Verification items for the finished model (mm, model axes). Face numbers are marked on the shaded views. A direction names the side the tool comes from. Give positions to 0.01 mm unless a question says otherwise; leave off trailing zeros. Loops run counter-clockwise (first coordinate to the right, second up) from the corner with the lowest first, then second, coordinate; pieces in that order, holes last. Notation, with made-up numbers: (77.5, -30) - (122.5, -30) arc R27 ccw to (122.5, 3) - close; hole circle Ø6 at (-25, 9). An arc over 180 degrees is marked (long way). Put each result on its own line as item: value. Start each with the question number.
```python
from build123d import *

# Parameters (mm, degrees)
SKETCH1_W            = 100
SKETCH1_H            = 16
BOSS_EXTRUDE1_DEPTH  = 3
SKETCH2_W            = 98
SKETCH2_H            = 14
CUT_EXTRUDE1_DEPTH   = 1
SKETCH5_W            = 20
SKETCH5_H            = 3
BOSS_EXTRUDE4_DEPTH  = 15
SKETCH6_W            = 20
SKETCH6_H            = 3
BOSS_EXTRUDE5_DEPTH  = 15
FILLET18_R           = 10
SKETCH7_W            = 3
SKETCH7_H            = 12
BOSS_EXTRUDE6_DEPTH  = 16
SKETCH8_W            = 6
SKETCH8_H            = 2
BOSS_EXTRUDE7_DEPTH  = 2
FILLET19_R           = 6
SKETCH10_W           = 60
SKETCH10_H           = 3
BOSS_EXTRUDE8_DEPTH  = 3
SKETCH11_W           = 60
SKETCH11_H           = 3
BOSS_EXTRUDE9_DEPTH  = 3
SKETCH12_W           = 0.95
SKETCH12_H           = 14
BOSS_EXTRUDE10_DEPTH = 3
SKETCH13_W           = 100
SKETCH13_H           = 0.95
BOSS_EXTRUDE11_DEPTH = 3
SKETCH14_W           = 0.95
SKETCH14_H           = 0.052088128
BOSS_EXTRUDE12_DEPTH = 3
SKETCH15_W           = 0.95
SKETCH15_H           = 0.047911872
SKETCH15_W_2         = 0.949734752
SKETCH15_H_2         = 0.052088128
BOSS_EXTRUDE13_DEPTH = 3
FILLET20_R           = 10
SKETCH17_W           = 98.1
SKETCH17_H           = 14.1
SKETCH17_W_2         = 97.1
SKETCH17_H_2         = 13.1
CUT_EXTRUDE2_DEPTH   = 4
SKETCH18_W           = 100
SKETCH18_H           = 16.05
SKETCH18_W_2         = 98
SKETCH18_H_2         = 14.05
CUT_EXTRUDE3_DEPTH   = 2


with BuildPart() as part:
    # Sketch1 → Boss-Extrude1 (new body)
    with BuildSketch(Plane(origin=(0, 0, 0), x_dir=(1, 0, 0), z_dir=(0, 1, 0))):
        with Locations((50, 8)):
            Rectangle(SKETCH1_W, SKETCH1_H)
    extrude(amount=BOSS_EXTRUDE1_DEPTH)

    # Sketch2 → Cut-Extrude1 (cut)
    with BuildSketch(Plane(origin=(0, 3, 0), x_dir=(1, 0, 0), z_dir=(0, 1, 0))):
        with Locations((50, 8)):
            Rectangle(SKETCH2_W, SKETCH2_H)
    extrude(amount=-CUT_EXTRUDE1_DEPTH, mode=Mode.SUBTRACT)

    # Sketch5 → Boss-Extrude4 (add)
    with BuildSketch(Plane.XY):
        with Locations((10, 1.5)):
            Rectangle(SKETCH5_W, SKETCH5_H)
        with Locations((90, 1.5)):
            Rectangle(SKETCH5_W, SKETCH5_H)
    extrude(amount=BOSS_EXTRUDE4_DEPTH)

    # Sketch6 → Boss-Extrude5 (add)
    with BuildSketch(Plane(origin=(0, 0, -16), x_dir=(-1, 0, 0), z_dir=(0, 0, -1))):
        with Locations((-90, 1.5)):
            Rectangle(SKETCH6_W, SKETCH6_H)
        with Locations((-10, 1.5)):
            Rectangle(SKETCH6_W, SKETCH6_H)
    extrude(amount=BOSS_EXTRUDE5_DEPTH)

    # Fillet18
    fillet18_edges = [part.edges().sort_by_distance(p)[0] for p in [
        (20, 1.5, 15),
        (0, 1.5, 15),
        (80, 1.5, 15),
        (100, 1.5, 15),
        (0, 1.5, -31),
        (20, 1.5, -31),
        (80, 1.5, -31),
        (100, 1.5, -31),
    ]]
    fillet(fillet18_edges, radius=FILLET18_R - 0.0001)  # a hair under: the kernel refuses the full size

    # Sketch7 → Boss-Extrude6 (add)
    with BuildSketch(Plane(origin=(0, 2, 0), x_dir=(1, 0, 0), z_dir=(0, 1, 0))):
        with Locations((95, 8)):
            Rectangle(SKETCH7_W, SKETCH7_H)
        with Locations((86, 8)):
            Rectangle(SKETCH7_W, SKETCH7_H)
        with Locations((77, 8)):
            Rectangle(SKETCH7_W, SKETCH7_H)
        with Locations((68, 8)):
            Rectangle(SKETCH7_W, SKETCH7_H)
        with Locations((59, 8)):
            Rectangle(SKETCH7_W, SKETCH7_H)
        with Locations((50, 8)):
            Rectangle(SKETCH7_W, SKETCH7_H)
        with Locations((41, 8)):
            Rectangle(SKETCH7_W, SKETCH7_H)
        with Locations((32, 8)):
            Rectangle(SKETCH7_W, SKETCH7_H)
        with Locations((23, 8)):
            Rectangle(SKETCH7_W, SKETCH7_H)
        with Locations((14, 8)):
            Rectangle(SKETCH7_W, SKETCH7_H)
        with Locations((5, 8)):
            Rectangle(SKETCH7_W, SKETCH7_H)
    extrude(amount=BOSS_EXTRUDE6_DEPTH)

    # Sketch8 → Boss-Extrude7 (add)
    with BuildSketch(Plane(origin=(0, 2, 0), x_dir=(1, 0, 0), z_dir=(0, 1, 0))):
        with Locations((90.5, 8)):
            Rectangle(SKETCH8_W, SKETCH8_H)
        with Locations((81.5, 8)):
            Rectangle(SKETCH8_W, SKETCH8_H)
        with Locations((72.5, 8)):
            Rectangle(SKETCH8_W, SKETCH8_H)
        with Locations((63.5, 8)):
            Rectangle(SKETCH8_W, SKETCH8_H)
        with Locations((54.5, 8)):
            Rectangle(SKETCH8_W, SKETCH8_H)
        with Locations((45.5, 8)):
            Rectangle(SKETCH8_W, SKETCH8_H)
        with Locations((36.5, 8)):
            Rectangle(SKETCH8_W, SKETCH8_H)
        with Locations((27.5, 8)):
            Rectangle(SKETCH8_W, SKETCH8_H)
        with Locations((18.5, 8)):
            Rectangle(SKETCH8_W, SKETCH8_H)
        with Locations((9.5, 8)):
            Rectangle(SKETCH8_W, SKETCH8_H)
    extrude(amount=BOSS_EXTRUDE7_DEPTH)

    # Fillet19
    fillet19_edges = [part.edges().sort_by_distance(p)[0] for p in [
        (95, 18, -2),
        (95, 18, -14),
        (86, 18, -2),
        (86, 18, -14),
        (77, 18, -2),
        (77, 18, -14),
        (68, 18, -2),
        (68, 18, -14),
        (59, 18, -2),
        (59, 18, -14),
        (50, 18, -2),
        (50, 18, -14),
        (41, 18, -2),
        (41, 18, -14),
        (32, 18, -2),
        (32, 18, -14),
        (23, 18, -14),
        (23, 18, -2),
        (14, 18, -2),
        (14, 18, -14),
        (5, 18, -2),
        (5, 18, -14),
    ]]
    fillet(fillet19_edges, radius=FILLET19_R - 0.0001)  # a hair under: the kernel refuses the full size

    # Sketch10 → Boss-Extrude8 (add)
    with BuildSketch(Plane(origin=(0, 0, -16), x_dir=(-1, 0, 0), z_dir=(0, 0, -1))):
        with Locations((-50, 1.5)):
            Rectangle(SKETCH10_W, SKETCH10_H)
    extrude(amount=BOSS_EXTRUDE8_DEPTH)

    # Sketch11 → Boss-Extrude9 (add)
    with BuildSketch(Plane.XY):
        with Locations((50, 1.5)):
            Rectangle(SKETCH11_W, SKETCH11_H)
    extrude(amount=BOSS_EXTRUDE9_DEPTH)

    # Sketch12 → Boss-Extrude10 (add)
    with BuildSketch(Plane(origin=(0, 3, 0), x_dir=(1, 0, 0), z_dir=(0, 1, 0))):
        with Locations((99.525, 7.997911872)):
            Rectangle(SKETCH12_W, SKETCH12_H)
        with Locations((0.475, 7.997911872)):
            Rectangle(SKETCH12_W, SKETCH12_H)
    extrude(amount=BOSS_EXTRUDE10_DEPTH)

    # Sketch13 → Boss-Extrude11 (add)
    with BuildSketch(Plane(origin=(0, 3, 0), x_dir=(1, 0, 0), z_dir=(0, 1, 0))):
        with Locations((50, 15.525)):
            Rectangle(SKETCH13_W, SKETCH13_H)
        with Locations((50, 0.475)):
            Rectangle(SKETCH13_W, SKETCH13_H)
    extrude(amount=BOSS_EXTRUDE11_DEPTH)

    # Sketch14 → Boss-Extrude12 (add)
    with BuildSketch(Plane(origin=(0, 3, 0), x_dir=(1, 0, 0), z_dir=(0, 1, 0))):
        with Locations((0.475, 15.023955936)):
            Rectangle(SKETCH14_W, SKETCH14_H)
    extrude(amount=BOSS_EXTRUDE12_DEPTH)

    # Sketch15 → Boss-Extrude13 (add)
    with BuildSketch(Plane(origin=(0, 3, 0), x_dir=(1, 0, 0), z_dir=(0, 1, 0))):
        with Locations((0.475, 0.973955936)):
            Rectangle(SKETCH15_W, SKETCH15_H)
        with Locations((99.525132624, 0.973955936)):
            Rectangle(SKETCH15_W_2, SKETCH15_H)
        with Locations((99.525, 15.023955936)):
            Rectangle(SKETCH15_W, SKETCH15_H_2)
    extrude(amount=BOSS_EXTRUDE13_DEPTH)

    # Fillet20
    fillet20_edges = [part.edges().sort_by_distance(p)[0] for p in [
        (20, 1.5, -19),
        (80, 1.5, -19),
        (80, 1.5, 3),
        (20, 1.5, 3),
    ]]
    fillet(fillet20_edges, radius=FILLET20_R)

    # Sketch17 → Cut-Extrude2 (cut)
    with BuildSketch(Plane(origin=(0, 6, 0), x_dir=(1, 0, 0), z_dir=(0, 1, 0))):
        with Locations((50, 8)):
            Rectangle(SKETCH17_W, SKETCH17_H)
        with Locations((50, 8)):
            Rectangle(SKETCH17_W_2, SKETCH17_H_2, mode=Mode.SUBTRACT)
    extrude(amount=-CUT_EXTRUDE2_DEPTH, mode=Mode.SUBTRACT)

    # Sketch18 → Cut-Extrude3 (cut)
    with BuildSketch(Plane(origin=(0, 6, 0), x_dir=(1, 0, 0), z_dir=(0, 1, 0))):
        with Locations((50, 7.975)):
            Rectangle(SKETCH18_W, SKETCH18_H)
        with Locations((50, 7.975)):
            Rectangle(SKETCH18_W_2, SKETCH18_H_2, mode=Mode.SUBTRACT)
    extrude(amount=-CUT_EXTRUDE3_DEPTH, mode=Mode.SUBTRACT)


solid = part.part
```
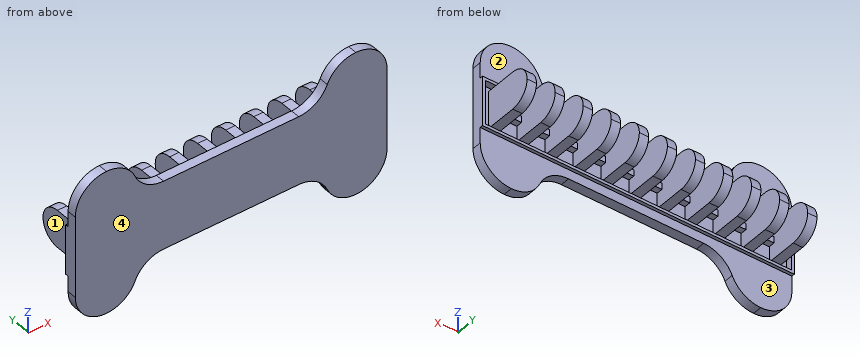
1) Section check A-A, the plane z = -27. Enter the section's corners in (x, y).
2) Depth check by flat-ended pin: P1, Ø8, axis at y = 16, z = -8.5, coming from the -X side; P2, Ø0.6, axis at x = 80.5, y = 3, coming from the -Z side; P3, Ø5, axis at x = 68, y = 9, coming from the -Z side; P4, Ø8, axis at y = 9, z = 5.5, coming from the -X side. Enter the tip coordinate at first touch or a pass-through.
3) Section check B-B, the plane x = 54. Enter the section's corners in (y, z), plus the area to 3 significant figures.
4) Set-up check for the marked faces 1, 2, 3 and 4: record each of +Z, -Z, +X, -X, +Y, -Y from which the full face is reachable in a straight line by a thin tool's end or side.
5) Section check D-D, the plane z = 1. Enter the section's corners in (x, y), plus the area to 3 significant figures.
6) Scan lines: line 1 along Y through (x, z) = (21, 6); line 2 along Y through (x, z) = (54.5, -8.5); line 3 along X through (y, z) = (1.25, -24). Record each from-to range of solid material in increasing order. Write a range as from..to.
7) Section check C-C, the plane y = 5.25. State how many separate pieces and enclosed holes the cut face has, plus the area to 3 significant figures.
Results are:
1. outline: (2, 0) - (18, 0) - (18, 3) - (2, 3) - close; (82, 0) - (98, 0) - (98, 3) - (82, 3) - close
2. P1: stops at x = 3.5
2. P2: stops at z = -24.92
2. P3: stops at z = -14
2. P4: passes through
3. outline: (0, -19) - (3, -19) - (3, -16) - (4, -16) - (4, -15.05) - (2, -15.05) - (2, -9) - (4, -9) - (4, -7) - (2, -7) - (2, -0.95) - (4, -0.95) - (4, 0) - (3, 0) - (3, 3) - (0, 3) - close
3. area: 57.8 mm2
4. face 1: +Y
4. face 2: +Z, +X, -X, +Y
4. face 3: -Z, +X, -X, +Y
4. face 4: +Z, -Z, +X, -X, -Y
5. outline: (0, 0) - (100, 0) - (100, 3) - (0, 3) - close
5. area: 300 mm2
6. line 1: y = 0..3
6. line 2: y = 0..4
6. line 3: x = 0.46..19.67, 80.33..99.54
7. separate pieces: 11
7. enclosed holes: 0
7. area: 396 mm2
